Read the model definition and answer for the solid it produces. Units are mm, in the model's axes. Round coordinates to 2 decimals unless told otherwise and drop trailing zeros. Use CSV: the item, a comma, the result in double quotes. Start each with the question number.
1. Given pin 1 Ø4 at (x, y) = (0, -25) entering from +Z; pin 2 Ø2 at (x, z) = (-19.5, 11.5) entering from -Y, each flat-ended and moving along its own axis, determine where each tip first touches the part or whether it passes through.
2. Determine the mould class of faces 1 (the conical face through (142.94, -142.71, 11.67)), 2 (the cylindrical face through (-133.52, 138.89, 6.44)), 3 (the flat face through (-2, -150, 4)), 4 (the conical face through (-142.94, 142.71, 11.67)) for opening direction X: +X half, -X half, draft (parallel to the pull), parting line (faces both ways), or undercut.
3. Consider line 1 along X through (y, z) = (65, 5.5); line 2 along Y through (x, z) = (134.5, 8.5). Determine where each line is inside the solid, lowest interval first.
from build123d import *

# Parameters (mm, degrees)
F0_W           = 300
F0_H           = 300
F1_DEPTH       = 12.7
F2_R           = 17.78
F3_SIZE        = 3.81
F5_D           = 9
F7_D           = 6.5278
F9_D           = 6.6
F9_CSINK_D     = 13.44
F9_CSINK_ANGLE = 90


with BuildPart() as f1:
    # F0 (on Top) → F1 (new body)
    with BuildSketch(Plane.XY):
        Rectangle(F0_W, F0_H)
    extrude(amount=F1_DEPTH)

    # F2
    f2_edges = [f1.edges().sort_by_distance(p)[0] for p in [
        (-150, -150, 6.35),
        (150, -150, 6.35),
        (150, 150, 6.35),
        (-150, 150, 6.35),
    ]]
    fillet(f2_edges, radius=F2_R)

    # F3
    f3_edges = [f1.edges().sort_by_distance(p)[0] for p in [
        (-150, 0, 12.7),
        (0, 150, 12.7),
        (150, 0, 12.7),
        (0, -150, 12.7),
        (144.792359, -144.792359, 12.7),
        (144.792359, 144.792359, 12.7),
        (-144.792359, -144.792359, 12.7),
        (-144.792359, 144.792359, 12.7),
    ]]
    chamfer(f3_edges, length=F3_SIZE)

    # F5 (through all)
    with Locations(Plane(origin=(0, 0, 0), x_dir=(1, 0, 0), z_dir=(0, 0, -1))):
        with Locations((-134.5, 134.5), (134.5, 134.5), (-134.5, -134.5), (134.5, -134.5)):
            Hole(F5_D / 2)

    # F7 (through all)
    with Locations(Plane(origin=(0, 0, 0), x_dir=(1, 0, 0), z_dir=(0, 0, -1))):
        with Locations((-65, 65), (65, 65), (65, -65), (-65, -65)):
            Hole(F7_D / 2)

    # F9 (through all)
    with Locations(Plane(origin=(0, 0, 0), x_dir=(1, 0, 0), z_dir=(0, 0, -1))):
        with Locations((0, 25), (25, 0), (0, -25), (-25, 0)):
            CounterSinkHole(F9_D / 2, F9_CSINK_D / 2, counter_sink_angle=F9_CSINK_ANGLE)


solid = f1.part
Filled sheet:
1,pin 1,"passes through"
1,pin 2,"stops at y = -148.39"
2,face 1,"+X half"
2,face 2,"undercut"
2,face 3,"draft"
2,face 4,"-X half"
3,line 1,"x = -150 to -68.26, -61.74 to 61.74, 68.26 to 150"
3,line 2,"y = -149.85 to -139, -130 to 130, 139 to 149.85"
